Source: CAD feature listing. Evaluate the final solid. Frame: model axes, mm. A direction names the side the tool comes from. Give positions to 0.01 mm unless a question says otherwise; leave off trailing zeros. Loops run counter-clockwise (first coordinate to the right, second up) from the corner with the lowest first, then second, coordinate; pieces in that order, holes last.
from build123d import *

# Parameters (mm, degrees)
BRIDA_BASE1_DEPTH          = 30
BRIDA_BASE1_DEPTH_BACK     = 30
BRIDA_DE_ARISTA1_DEPTH     = 60
CORTAR_EXTRUIR4_DEPTH      = 207.650630806
CORTAR_EXTRUIR4_DEPTH_BACK = 207.650630806
CROQUIS13_W                = 32
CROQUIS13_H                = 40
REDONDEO1_R                = 10
SALIENTE_EXTRUIR1_DEPTH    = 20
REDONDEO2_R                = 5
CORTAR_EXTRUIR5_REACH      = 213.826
CROQUIS18_R                = 3.5
REDONDEO3_R                = 5


# Sheet-metal steps are written as plain solids
with BuildPart() as part:
    # Croquis2 → Brida base1 (new, two sides: drawn at the far end of the back side and taken through both)
    with BuildSketch(Plane.XY.offset(-BRIDA_BASE1_DEPTH_BACK)):
        with BuildLine():
            ThreePointArc((0, 0), (54.558363857, 88.248906187), (55, 192))
            Line((55, 192), (59.586947027, 193.271816408))
            ThreePointArc((59.586947027, 193.271816408), (59.134317403, 86.938086161), (3.217852989, -3.507566413))
            Line((3.217852989, -3.507566413), (0, 0))
        make_face()
    extrude(amount=BRIDA_BASE1_DEPTH + BRIDA_BASE1_DEPTH_BACK)

    # Brida de arista1 section (across the edge) → Brida de arista1 (add)
    with BuildSketch(Plane(origin=(2.413685543, -4.245312279, 30), x_dir=(0.6751606504214892, 0.7376707233735331, 0), z_dir=(0, 0, -1))):
        with BuildLine():
            Line((-4.76, 1.091308501), (-4.76, 22.805371535))
            Line((-4.76, 22.805371535), (0, 22.805371535))
            Line((0, 22.805371535), (0, 1.091308501))
            ThreePointArc((0, 1.091308501), (0.324409792, 0.354031164), (1.087155743, 0.095113803))
            Line((1.087155743, 0.095113803), (1.502017078, -4.64677296))
            ThreePointArc((1.502017078, -4.64677296), (-2.891399596, -3.155408959), (-4.76, 1.091308501))
        make_face()
    extrude(amount=BRIDA_DE_ARISTA1_DEPTH)

    # Croquis13 → Cortar-Extruir4 (cut, two sides: drawn at the far end of the back side and taken through both)
    with BuildSketch(Plane(origin=(0, 0, 0), x_dir=(0, 0, -1), z_dir=(1, 0, 0)).offset(-CORTAR_EXTRUIR4_DEPTH_BACK)):
        Polygon((-10, 193.271816408), (-30, 8.271816408), (-30, 193.271816408), align=None)
        Polygon((30, 193.271816408), (10, 193.271816408), (30, 8.271816408), align=None)
        with Locations((0, 28)):
            Rectangle(CROQUIS13_W, CROQUIS13_H)
    extrude(amount=CORTAR_EXTRUIR4_DEPTH + CORTAR_EXTRUIR4_DEPTH_BACK, mode=Mode.SUBTRACT)

    # Redondeo1
    redondeo1_edges = [part.edges().sort_by_distance(p)[0] for p in [
        (57.293473513, 192.635908204, 10.068746833),
        (57.293473513, 192.635908204, -10.068746833),
    ]]
    fillet(redondeo1_edges, radius=REDONDEO1_R)

    # Croquis17 → Saliente-Extruir1 (add)
    with BuildSketch(Plane(origin=(0, 0, -30), x_dir=(-1, 0, 0), z_dir=(0, 0, -1))):
        Polygon((-16.022775764, -23.1539144), (-0.004947179, -8.493433479), (-3.218711875, -4.982120836), (-19.23654046, -19.642601757), align=None)
    saliente_extruir1 = extrude(amount=SALIENTE_EXTRUIR1_DEPTH)

    # Simetría1: Saliente-Extruir1 across plane
    add(saliente_extruir1.mirror(Plane.XY))

    # Redondeo2
    redondeo2_edges = [part.edges().sort_by_distance(p)[0] for p in [
        (17.629658112, -21.398258079, -50),
        (1.611829527, -6.737777158, -50),
        (17.629658112, -21.398258079, 50),
        (1.611829527, -6.737777158, 50),
    ]]
    fillet(redondeo2_edges, radius=REDONDEO2_R)

    # Croquis18 → Cortar-Extruir5 (cut, up to next)
    with BuildSketch(Plane(origin=(-1.014102827, -1.107994025, 0), x_dir=(0, 0, -1), z_dir=(0.6751606504214892, 0.7376707233735331, 0)), mode=Mode.PRIVATE) as cortar_extruir5_sk1:
        with Locations(Location((30, -13.952144495, 0), (0, 0, 90))):
            Circle(CROQUIS18_R)
    cortar_extruir5_tool1 = extrude(cortar_extruir5_sk1.sketch, amount=-CORTAR_EXTRUIR5_REACH, mode=Mode.PRIVATE) & part.part
    # Croquis18 → Cortar-Extruir5 (cut, up to next)
    with BuildSketch(Plane(origin=(-1.014102827, -1.107994025, 0), x_dir=(0, 0, -1), z_dir=(0.6751606504214892, 0.7376707233735331, 0)), mode=Mode.PRIVATE) as cortar_extruir5_sk2:
        with Locations(Location((-30, -13.952144495, 0), (0, 0, 270))):
            Circle(CROQUIS18_R)
    cortar_extruir5_tool2 = extrude(cortar_extruir5_sk2.sketch, amount=-CORTAR_EXTRUIR5_REACH, mode=Mode.PRIVATE) & part.part
    add(cortar_extruir5_tool1.solids().sort_by_distance((9.277986, -10.527933, -30))[0], mode=Mode.SUBTRACT)
    add(cortar_extruir5_tool2.solids().sort_by_distance((9.277986, -10.527933, 30))[0], mode=Mode.SUBTRACT)

    # Redondeo3
    redondeo3_edges = [part.edges().sort_by_distance(p)[0] for p in [
        (40.577357411, 48, -16),
        (11.485461299, 8, -16),
        (11.485461299, 8, 16),
        (40.577357411, 48, 16),
    ]]
    fillet(redondeo3_edges, radius=REDONDEO3_R)


solid = part.part
1) Contact query for flat-ended pins moving along their axis: P1, Ø12, axis at x = 17.5, z = -4, coming from the +Y side; P2, Ø5, axis at x = 5, y = -4, coming from the -Z side; P3, Ø1, axis at x = 42, z = -23.5, coming from the -Y side; P4, Ø5, axis at x = 9.5, y = -3, coming from the +Z side. Output: stop coordinate, or through.
Checks:
P1: stops at y = 8
P2: stops at z = -49.17
P3: stops at y = 44.75
P4: passes through
2) Cut plane C-C (x = 53). Return loops of the section in (y, z), and give its area (3 significant figures).
Checks:
outline: (68.89, -23.45) - (83.09, -21.91) - (83.09, 21.91) - (68.89, 23.45) - close
area: 644 mm2
3) Cut plane A-A (y = 32). Return loops of the section in (x, z), and give its area (3 significant figures).
Checks:
outline: (27.91, -27.43) - (33.67, -27.43) - (33.67, -16) - (27.91, -16) - close; (27.91, 16) - (33.67, 16) - (33.67, 27.43) - (27.91, 27.43) - close
area: 132 mm2
4) Cut plane B-B (z = 18.5). Return loops of the section in (x, y), and give its area (3 significant figures).
Checks:
outline: (0, -8.49) - (16.02, -23.15) - (19.24, -19.64) - (3.22, -4.98) arc R1 cw to (3.22, -3.51) arc R195.98 ccw to (64.94, 114.65) - (60.14, 114.65) arc R191.22 cw to (0, 0) arc R5.76 ccw to start
area: 768 mm2
5) Pull-direction query (X, two-part tool) for faces 1 (the cylindrical face through (16.555, -20.46, -48.496)), 2 (the cylindrical face through (39, 47, -14)), 3 (the cylindrical face through (7.36, -11.95, 26.53)); classes: released by +X, released by -X, zero draft, split by the parting line, or undercut.
Checks:
face 1: released by +X
face 2: zero draft
face 3: undercut
6) Reachability of faces 4 (the cylindrical face through (39, 47, 14)), 5 (the cylindrical face through (13, 10, -15)), 6 (the cylindrical face through (16.555, -20.46, 48.496)), 7 (the flat face through (56.87, 90.31, 21.13)), 8 (the flat face through (6, 2, -30)) from +Z, -Z, +X, -X, +Y, -Y: full face, straight path, thin tool, end or side. Return the list, or none.
Checks:
face 4: +X, -X, -Y
face 5: +X, -X, +Y
face 6: +Z, +X, -Y
face 7: +Z, +X, -X, +Y
face 8: -Z, -X, +Y
7) Ray query, probe 1 along Y at (x, z) = (3, -13.5); probe 2 along X at (y, z) = (140.5, -7.5); probe 3 along X at (y, z) = (5, 26). Return the intervals inside material, ascending.
Checks:
probe 1: y = -11.23 to -4.69, -3.8 to 2.81
probe 2: x = 61.95 to 66.71
probe 3: x = 5.25 to 11.93
8) Cut plane D-D (y = 123.5). Return loops of the section in (x, z).
Checks:
outline: (61.16, -17.54) - (65.94, -17.54) - (65.94, 17.54) - (61.16, 17.54) - close
